For this review, take the finished solid that the model builds, in its own axes (mm). A direction names the side the tool comes from. Coordinates: 2 decimals unless noted, no trailing zeros. Loops run counter-clockwise (first coordinate to the right, second up) from the corner with the lowest first, then second, coordinate; pieces in that order, holes last. Notation, with made-up numbers: (56, 58.25) - (95, 58.25) arc R21 ccw to (95, 79.25) - close; hole circle Ø9 at (53, 18). An arc over 180 degrees is marked (long way). Use one line per item in the form item = value. Start each with the question number.
1. Add section B-B on x = -45. Give the boundary of the cut face in (y, z).
2. Draft analysis for pull direction X (two halves, no side actions). For faces 1 (the face through (-1.7, 84.3, 0.8)), 2 (the face through (-86.71, 91.05, 0.79)), 3 (the face through (5.579, 4.854, 0.789)), 4 (the face through (-2.77, 8.54, 0.81)), state which applies: +X half, -X half, draft (parallel to the pull), parting line (faces both ways), or undercut.
3. Machinability: for faces 5 (the face through (-77.7, 84.3, 0.8)), 6 (the face through (-70.66, 13.1, 0.81)), which of the approach directions +Z, -Z, +X, -X, +Y, -Y give a long, thin tool a straight path to every point of the face, cutting with its end or side? Answer none if there is none.
4. To check wall thickness, follow probe 1 along X at (y, z) = (82, 0.95); probe 2 along Y at (x, z) = (-51, 0.55); probe 3 along X at (y, z) = (13, 0.4). State the ranges of each line that lie inside material, in increasing order.
5. For pin 1 Ø2.5 at (x, y) = (-2.57, 82.95) entering from -Z; pin 2 Ø4 at (x, y) = (-78.57, 82.95) entering from +Z; pin 3 Ø0.5 at (x, z) = (-36.5, 1) entering from -Y, all flat-tipped, find the tip position at first contact; note any pin that passes through.
6. Add section A-A on z = 0.4. Count the separate pieces of the cut face and the enclosed holes in it, and give its area (3 significant figures).
```python
from build123d import *

# Parameters (mm, degrees)
SKETCH1_R                  = 0.5
BOSS_EXTRUDE1_DEPTH        = 1.6
F_3_2_3_2_DIAMETER_HOLE3_D = 3.2
FILLET1_R                  = 3
FILLET2_R                  = 1


with BuildPart() as part:
    # Sketch1 → Boss-Extrude1 (new body)
    with BuildSketch(Plane.XY):
        with BuildLine():
            Line((-55.56534388, 7.95185693), (-55.56534388, 13.95185693))
            Line((-55.56534388, 13.95185693), (-71.56534388, 13.95185693))
            Line((-71.56534388, 13.95185693), (-71.56534388, 3.95185693))
            Line((-71.56534388, 3.95185693), (-84.56534388, 3.95185693))
            ThreePointArc((-84.56534388, 3.95185693), (-86.686664224, 4.830536587), (-87.56534388, 6.95185693))
            Line((-87.56534388, 6.95185693), (-87.56534388, 88.95185693))
            ThreePointArc((-87.56534388, 88.95185693), (-86.686664224, 91.073177274), (-84.56534388, 91.95185693))
            Line((-84.56534388, 91.95185693), (3.43465612, 91.95185693))
            ThreePointArc((3.43465612, 91.95185693), (5.555976464, 91.073177274), (6.43465612, 88.95185693))
            Line((6.43465612, 88.95185693), (6.43465612, 6.95185693))
            ThreePointArc((6.43465612, 6.95185693), (5.555976464, 4.830536587), (3.43465612, 3.95185693))
            Line((3.43465612, 3.95185693), (-24.56534388, 3.95185693))
            Line((-24.56534388, 3.95185693), (-24.56534388, 7.95185693))
            Line((-24.56534388, 7.95185693), (-55.56534388, 7.95185693))
        make_face()
        with Locations((-59.10534388, 18.75185693)):
            Circle(SKETCH1_R, mode=Mode.SUBTRACT)
        with Locations((-64.18534388, 18.75185693)):
            Circle(SKETCH1_R, mode=Mode.SUBTRACT)
    extrude(amount=BOSS_EXTRUDE1_DEPTH)

    # Ø3.2 (3.2) Diameter Hole3 (through all)
    with Locations(Plane(origin=(0, 0, 0), x_dir=(-1, 0, 0), z_dir=(0, 0, -1))):
        with Locations((78.56534388, 6.95185693), (78.56534388, 82.95185693), (2.56534388, 82.95185693), (2.56534388, 6.95185693)):
            Hole(F_3_2_3_2_DIAMETER_HOLE3_D / 2)

    # Fillet1
    fillet1_edges = [part.edges().sort_by_distance(p)[0] for p in [
        (-24.56534388, 7.95185693, 0.8),
        (-55.56534388, 13.95185693, 0.8),
        (-71.56534388, 13.95185693, 0.8),
    ]]
    fillet(fillet1_edges, radius=FILLET1_R)

    # Fillet2
    fillet2_edges = [part.edges().sort_by_distance(p)[0] for p in [
        (-24.56534388, 3.95185693, 0.8),
        (-71.56534388, 3.95185693, 0.8),
        (-55.56534388, 7.95185693, 0.8),
    ]]
    fillet(fillet2_edges, radius=FILLET2_R - 0.0001)  # a hair under: the kernel refuses the full size


solid = part.part
```
Conclusion:
q1.outline = (7.95, 0) - (91.95, 0) - (91.95, 1.6) - (7.95, 1.6) - close
q2.face_1 = undercut
q2.face_2 = -X half
q2.face_3 = +X half
q2.face_4 = undercut
q3.face_5 = +Z, -Z
q3.face_6 = +Z, -Z, -Y
q4.probe_1 = -87.57 to -79.85, -77.28 to -3.85, -1.28 to 6.43
q4.probe_2 = 7.95 to 91.95
q4.probe_3 = -87.57 to -70.76, -56.37 to 6.43
q5.pin_1 = through
q5.pin_2 = 1.6
q5.pin_3 = 7.95
q6.separate_pieces = 1
q6.enclosed_holes = 6
q6.area = 7,950 mm^2
